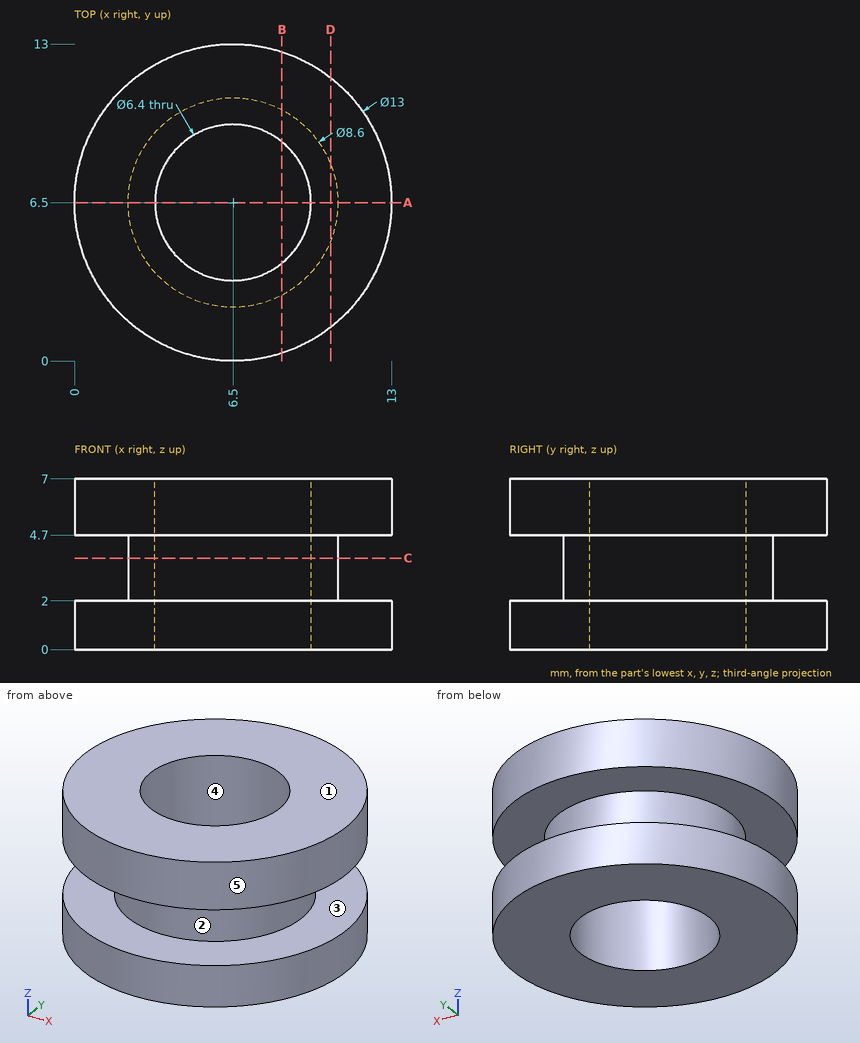
Geometry check sheet. Reference: drawing and pictorial views, mm from the part's lowest x, y, z. A direction names the side the tool comes from. Coordinates: 2 decimals unless noted, no trailing zeros. Order: outer loops, then holes, each group sorted by start corner. A loop starts at its lowest first (then second) coordinate and runs counter-clockwise, first axis right, second up. Notation, with made-up numbers: (76, -33.75) - (106, -33.75) arc R13 ccw to (106, -18.75) - close; hole circle Ø4 at (42.5, 11.25). An arc over 180 degrees is marked (long way). Answer in a Markdown table with one row per item. Add a question column.
1) Cross-section at C-C, the plane z = 3.75. Record the cut outline in (x, y).
2) Set-up check for the marked faces 1 and 2: record each of +Z, -Z, +X, -X, +Y, -Y from which the full face is reachable in a straight line by a thin tool's end or side.
3) Cross-section at D-D, the plane x = 10.5. Record the cut outline in (y, z).
4) Gauge pin test, flat ends, axial feed: P1, Ø2, axis at x = 11, z = 6, coming from the -Y side; P2, Ø2, axis at x = 9.5, z = 4, coming from the -Y side; P3, Ø1, axis at y = 10.5, z = 6, coming from the -X side; P4, Ø1.5, axis at x = 6, z = 5, coming from the +Y side. Record the tip position at first contact, or that the pin passes through.
5) Release check for a two-part mould opening along Y. For the marked faces 3, 4 and 5 record: +Y half, -Y half, draft (parallel to the pull), parting line (faces both ways), or undercut.
6) Material ranges on line 1 along Y through (x, z) = (6.5, 5); line 2 along Z through (x, y) = (1.75, 6); line 3 along Y through (x, z) = (6.5, 4.5), recorded low to high. Write a range as [from, to].
7) Cross-section at B-B, the plane x = 8.5. Record the cut outline in (y, z).
8) Cross-section at A-A, the plane y = 6.5. Record the cut outline in (x, z).
Check result:
| question | item | result |
|---|---|---|
| 1 | outline | circle Ø8.6 at (6.5, 6.5); hole circle Ø6.4 at (6.5, 6.5) |
| 2 | face 1 | +Z, +X, -X, +Y, -Y |
| 2 | face 2 | none |
| 3 | outline | (1.38, 0) - (11.62, 0) - (11.62, 2) - (8.08, 2) - (8.08, 4.7) - (11.62, 4.7) - (11.62, 7) - (1.38, 7) - (1.38, 4.7) - (4.92, 4.7) - (4.92, 2) - (1.38, 2) - close |
| 4 | P1 | stops at y = 1.02 |
| 4 | P2 | stops at y = 0.42 |
| 4 | P3 | stops at x = 1.02 |
| 4 | P4 | stops at y = 13 |
| 5 | face 3 | draft |
| 5 | face 4 | undercut |
| 5 | face 5 | parting line |
| 6 | line 1 | y = [0, 3.3], [9.7, 13] |
| 6 | line 2 | z = [0, 2], [4.7, 7] |
| 6 | line 3 | y = [2.2, 3.3], [9.7, 10.8] |
| 7 | outline | (0.32, 0) - (4, 0) - (4, 7) - (0.32, 7) - (0.32, 4.7) - (2.69, 4.7) - (2.69, 2) - (0.32, 2) - close; (9, 0) - (12.68, 0) - (12.68, 2) - (10.31, 2) - (10.31, 4.7) - (12.68, 4.7) - (12.68, 7) - (9, 7) - close |
| 8 | outline | (0, 0) - (3.3, 0) - (3.3, 7) - (0, 7) - (0, 4.7) - (2.2, 4.7) - (2.2, 2) - (0, 2) - close; (9.7, 0) - (13, 0) - (13, 2) - (10.8, 2) - (10.8, 4.7) - (13, 4.7) - (13, 7) - (9.7, 7) - close |
